Model file for the job. Use its own axes, mm. A direction names the side the tool comes from. Give positions to 0.01 mm unless a question says otherwise; leave off trailing zeros. Loops run counter-clockwise (first coordinate to the right, second up) from the corner with the lowest first, then second, coordinate; pieces in that order, holes last. Notation, with made-up numbers: M 60.5,-18 L 96.5,-18 A18 cw 96.5,3 Z; hole C -23.5,55 d11. An arc over 180 degrees is marked long. Answer in a Markdown table with one row per item.
```python
from build123d import *

# Parameters (mm, degrees)
F0_W     = 60
F0_H     = 40
F1_DEPTH = 40
F2_W     = 40
F2_H     = 40
F3_DEPTH = 20
F5_DEPTH = 10


with BuildPart() as f1:
    # F0 (on Front) → F1 (new body)
    with BuildSketch(Plane.XZ):
        with Locations((30, 20)):
            Rectangle(F0_W, F0_H)
    extrude(amount=F1_DEPTH)

    # F2 (on face) → F3 (cut)
    with BuildSketch(Plane.XY.offset(40)):
        with Locations((40, -20)):
            Rectangle(F2_W, F2_H)
    extrude(amount=-F3_DEPTH, mode=Mode.SUBTRACT)

    # F4 (on face) → F5 (cut)
    with BuildSketch(Plane.XY.offset(20)):
        with BuildLine():
            Line((60, 0), (40, 0))
            ThreePointArc((40, 0), (45.358984, -20), (40, -40))
            Line((40, -40), (60, -40))
            Line((60, -40), (60, 0))
        make_face()
    extrude(amount=-F5_DEPTH, mode=Mode.SUBTRACT)


solid = f1.part
```
Q1. Drop flat-ended pins along their axis: pin 1 (3 mm diameter, centred on y = -29.5, z = 5, fed in from -X); pin 2 (2 mm diameter, centred on x = 53, y = -24, fed in from +Z); pin 3 (6 mm diameter, centred on y = -24.5, z = 25.5, fed in from +X); pin 4 (12.5 mm diameter, centred on x = 30.5, y = -27.5, fed in from +Z). Give the stop position or say it passes through.
Reported:
| item | result |
|---|---|
| pin 1 | x = 0 |
| pin 2 | z = 10 |
| pin 3 | x = 20 |
| pin 4 | z = 20 |
Q2. Probe probe 1 along Z at (x, y) = (37.5, -18.5); probe 2 along Z at (x, y) = (47.5, -3.5). List the from-to ranges inside material, lowest first.
Reported:
| item | result |
|---|---|
| probe 1 | 0 to 20 |
| probe 2 | 0 to 10 |
Q3. Saw through at C-C (z = 34). Give the cut face in (x, y).
Reported:
| item | result |
|---|---|
| outline | M 0,-40 L 20,-40 L 20,0 L 0,0 Z |
Q4. Saw through at A-A (y = -6). Give the cut face in (x, z).
Reported:
| item | result |
|---|---|
| outline | M 0,0 L 60,0 L 60,10 L 42.83,10 L 42.83,20 L 20,20 L 20,40 L 0,40 Z |
Q5. Saw through at D-D (y = -36.5). Give the cut face in (x, z), and give its area (3 significant figures).
Reported:
| item | result |
|---|---|
| outline | M 0,0 L 60,0 L 60,10 L 41.8,10 L 41.8,20 L 20,20 L 20,40 L 0,40 Z |
| area | 1,420 mm² |
Q6. Saw through at B-B (x = 52). Give the cut face in (y, z), and give its area (3 significant figures).
Reported:
| item | result |
|---|---|
| outline | M -40,0 L 0,0 L 0,10 L -40,10 Z |
| area | 400 mm² |
Q7. 3-axis set-ups, long thin cutter, end or side, ignore diameter. For faces 1 (the face through (33, -20, 20)), 2 (the face through (10, -20, 40)), 3 (the face through (45.358, -19.707, 15.07)): which of +Z, -Z, +X, -X, +Y, -Y reach the whole face in a straight line?
Reported:
| item | result |
|---|---|
| face 1 | +Z, +X, +Y, -Y |
| face 2 | +Z, +X, -X, +Y, -Y |
| face 3 | +Z, +X |
